For this review, use the dimensioned drawing (mm, ordinates from the lowest corner) and the shaded views. A direction names the side the tool comes from. Give positions to 0.01 mm unless a question says otherwise; leave off trailing zeros. Write each loop counter-clockwise with the first axis right and the second up, starting at its lowest first coordinate (ties: lowest second). Pieces come first, ordered by that corner, then holes. Notation, with made-up numbers: (-10.75, 85) -> (1.25, 85) arc R15 cw to (1.25, 97) -> close; hole circle Ø1 at (-3.75, 21). An arc over 180 degrees is marked (long way). Return JSON: item names as keys, results as strings.
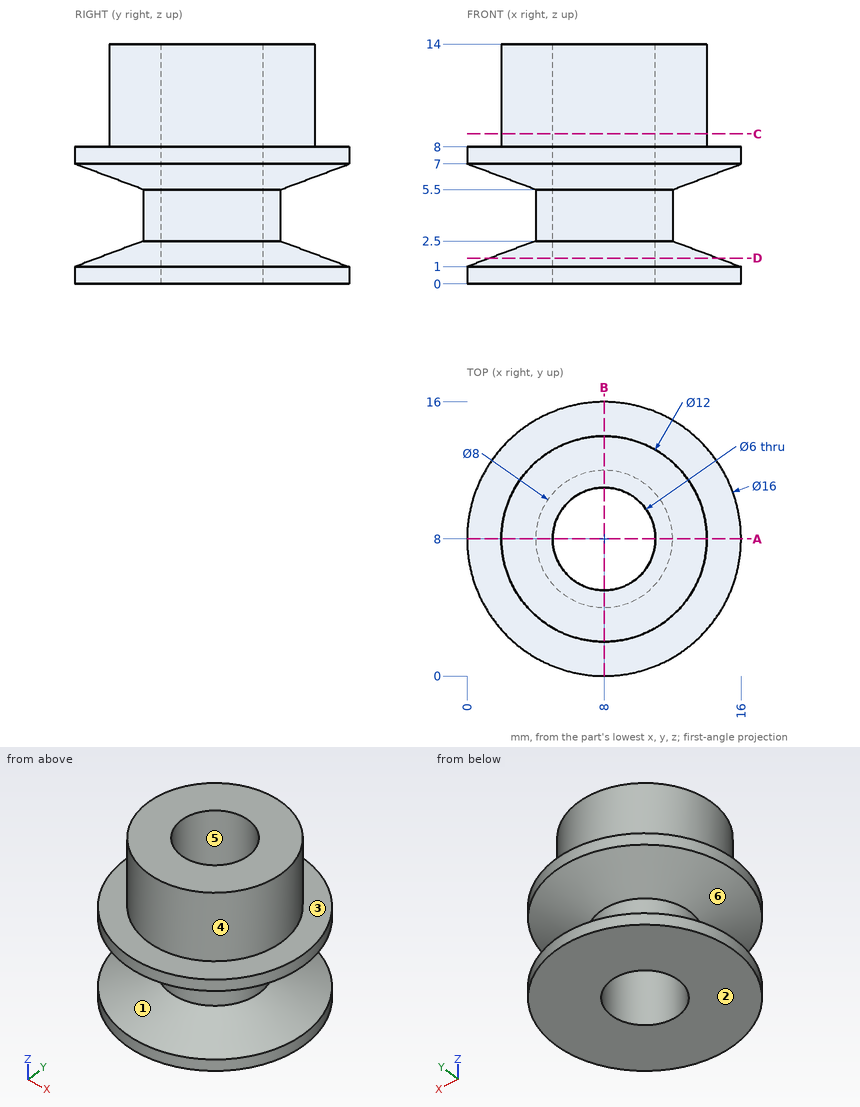
1. To check wall thickness, follow probe 1 along Y at (x, z) = (8, 3.25); probe 2 along Y at (x, z) = (8, 7.75); probe 3 along X at (y, z) = (8, 9.75). State the ranges of each line that lie inside material, in increasing order.
Results found:
{"probe 1": "y = 4 to 5, 11 to 12", "probe 2": "y = 0 to 5, 11 to 16", "probe 3": "x = 2 to 5, 11 to 14"}
2. Add section A-A, the plane y = 8. State the section outline as (x, z) points.
Results found:
{"outline": "(0, 0) -> (5, 0) -> (5, 14) -> (2, 14) -> (2, 8) -> (0, 8) -> (0, 7) -> (4, 5.5) -> (4, 2.5) -> (0, 1) -> close; (11, 0) -> (16, 0) -> (16, 1) -> (12, 2.5) -> (12, 5.5) -> (16, 7) -> (16, 8) -> (14, 8) -> (14, 14) -> (11, 14) -> close"}
3. Add section C-C, the plane z = 8.75. State the section outline as (x, y) points, plus the area to 3 significant figures.
Results found:
{"outline": "circle Ø12 at (8, 8); hole circle Ø6 at (8, 8)", "area": "84.8 mm²"}
4. For pin 1 (2 mm diameter, centred on x = 3, z = 6.5, fed in from +Y); pin 2 (3.5 mm diameter, centred on x = 8, y = 8, fed in from -Z); pin 3 (2 mm diameter, centred on y = 11.5, z = 7, fed in from +X), all flat-tipped, find the tip position at first contact; note any pin that passes through.
Results found:
{"pin 1": "stops at y = 14.85", "pin 2": "passes through", "pin 3": "stops at x = 15.6"}
5. Add section D-D, the plane z = 1.5. State the section outline as (x, y) points.
Results found:
{"outline": "circle Ø13.33 at (8, 8); hole circle Ø6 at (8, 8)"}
6. For the marked faces 5 and 6, list the 3-axis set-ups (+Z, -Z, +X, -X, +Y, -Y) from which the entire face can be reached by the end or side of a thin tool; tool diameter is ignored.
Results found:
{"face 5": "+Z, -Z", "face 6": "none"}
7. The part is to be moulded in two halves that separate along Z. For the marked faces 1, 2, 3 and 4, say which applies: +Z half, -Z half, draft (parallel to the pull), parting line (faces both ways), or undercut.
Results found:
{"face 1": "undercut", "face 2": "-Z half", "face 3": "+Z half", "face 4": "draft"}
